The model under review builds one solid part; all positions refer to its coordinate system, in mm. Face numbers are marked on the shaded views. A direction names the side the tool comes from. Round coordinates to 2 decimals unless told otherwise and drop trailing zeros. Write each loop counter-clockwise with the first axis right and the second up, starting at its lowest first coordinate (ties: lowest second). Pieces come first, ordered by that corner, then holes. Notation, with made-up numbers: (72.5, 70.25) - (95.5, 70.25) arc R15 cw to (95.5, 94.25) - close; hole circle Ø9 at (84, 89.5). An arc over 180 degrees is marked (long way). Write each question's results on one line, items separated by ' | '.
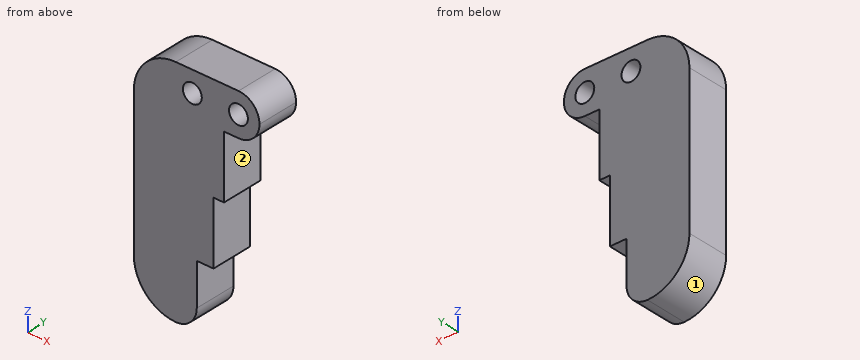
```python
from build123d import *

# Parameters (mm, degrees)
BOSS_EXTRUDE1_DEPTH = 10
SKETCH3_R           = 2.25
CUT_EXTRUDE1_DEPTH  = 10
FILLET1_R           = 10
FILLET2_R           = 5


with BuildPart() as part:
    # Sketch2 → Boss-Extrude1 (new body)
    with BuildSketch(Plane(origin=(0, 0, 0), x_dir=(1, 0, 0), z_dir=(0, 1, 0))):
        Polygon((-8.45, 15), (-8.45, 0), (0, 0), (0, -10), (-29.95, -10), (-29.95, 45), (-14.95, 45), (-14.95, 30), (-10.95, 30), (-10.95, 15), align=None)
    extrude(amount=BOSS_EXTRUDE1_DEPTH)

    # Sketch3 → Cut-Extrude1 (cut)
    with BuildSketch(Plane(origin=(0, 10, 0), x_dir=(1, 0, 0), z_dir=(0, 1, 0))):
        with Locations(Location((-16, -5, 0), (0, 0, 270))):
            Circle(SKETCH3_R)
        with Locations(Location((-5, -5, 0), (0, 0, 270))):
            Circle(SKETCH3_R)
    extrude(amount=-CUT_EXTRUDE1_DEPTH, mode=Mode.SUBTRACT)

    # Fillet1
    fillet1_edges = [part.edges().sort_by_distance(p)[0] for p in [
        (-29.95, 5, 10),
        (-29.95, 5, -45),
    ]]
    fillet(fillet1_edges, radius=FILLET1_R)

    # Fillet2
    fillet2_edges = [part.edges().sort_by_distance(p)[0] for p in [
        (-14.95, 5, -45),
        (0, 5, 0),
        (0, 5, 10),
    ]]
    fillet(fillet2_edges, radius=FILLET2_R - 0.0001)  # a hair under: the kernel refuses the full size


solid = part.part
```
Q1. Tool access review of the marked faces 1 and 2: name each direction out of +Z, -Z, +X, -X, +Y, -Y from which nothing blocks a thin tool from reaching the whole face with its end or side.
Evaluation:
face 1: -Z, -X, +Y, -Y | face 2: -Z, +X, +Y, -Y
Q2. We need section D-D (x = -16). State the section outline as (y, z) points.
Evaluation:
outline: (0, -43.07) - (10, -43.07) - (10, 2.75) - (0, 2.75) - close; (0, 7.25) - (10, 7.25) - (10, 10) - (0, 10) - close
Q3. We need section B-B (x = -6). State the section outline as (y, z) points, plus the area to 3 significant figures.
Evaluation:
outline: (0, 0) - (10, 0) - (10, 2.98) - (0, 2.98) - close; (0, 7.02) - (10, 7.02) - (10, 10) - (0, 10) - close | area: 59.7 mm^2
Q4. We need section A-A (y = 5.75). State how many separate pieces and enclosed holes the cut face has, plus the area to 3 significant figures.
Evaluation:
separate pieces: 1 | enclosed holes: 2 | area: 1,040 mm^2
Q5. For probe 1 along X at (y, z) = (3.75, 5); probe 2 along X at (y, z) = (3.5, 6); probe 3 along X at (y, z) = (4.75, -16), list the stretches that pass through material, from the lowest coordinate up.
Evaluation:
probe 1: x = -28.61 to -18.25, -13.75 to -7.25, -2.75 to 0 | probe 2: x = -27.95 to -18.02, -13.98 to -7.02, -2.98 to -0.1 | probe 3: x = -29.95 to -10.95
Q6. Insertion check: P1, Ø3, axis at y = 3.5, z = -4, coming from the +X side; P2, Ø2, axis at y = 7.5, z = -25.5, coming from the +X side; P3, Ø6, axis at x = -4, y = 8.5, coming from the -Z side. Each pin has a flat end and moves straight along its axis. Give the tip position at first contact, or say it passes through.
Evaluation:
P1: stops at x = -8.45 | P2: stops at x = -10.95 | P3: stops at z = 0
Q7. We need section C-C (z = -24.5). State the section outline as (x, y) points.
Evaluation:
outline: (-29.95, 0) - (-10.95, 0) - (-10.95, 10) - (-29.95, 10) - close
